Geometry check sheet. Reference: drawing and pictorial views, mm from the part's lowest x, y, z. Coordinates: 2 decimals unless noted, no trailing zeros. Order: outer loops, then holes, each group sorted by start corner. A loop starts at its lowest first (then second) coordinate and runs counter-clockwise, first axis right, second up. Notation, with made-up numbers: M 48,51.5 L 60,51.5 A8 ccw 60,55.5 Z; hole C 9.5,42.25 d7. An arc over 180 degrees is marked long. Return JSON: item names as keys, results as strings.
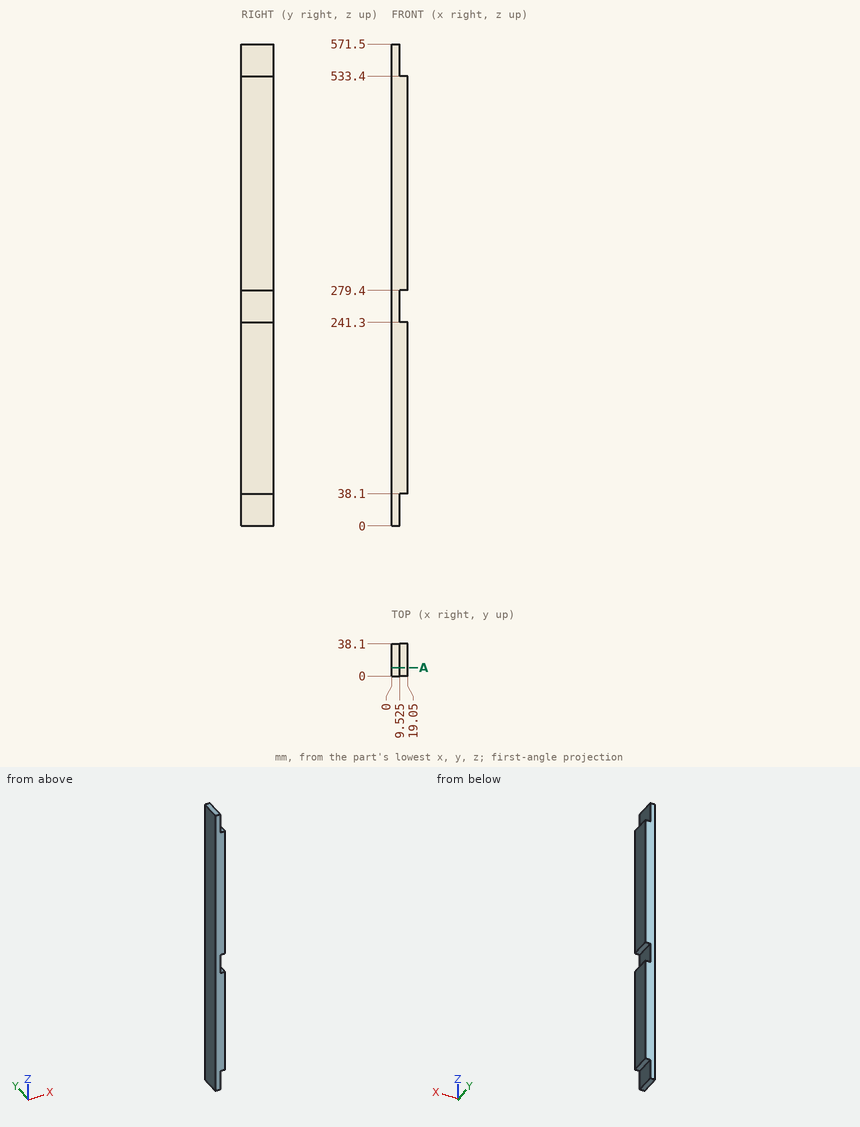
Q1. Cross-section at A-A, the plane y = 10. Record the boundary of the cut face in (x, z) (3 decimals).
Values:
{"outline": "M 0,0 L 9.525,0 L 9.525,38.1 L 19.05,38.1 L 19.05,241.3 L 9.525,241.3 L 9.525,279.4 L 19.05,279.4 L 19.05,533.4 L 9.525,533.4 L 9.525,571.5 L 0,571.5 Z"}
Q2. Go/stop test with flat-tipped pins: pin 1 (11.5 mm diameter, centred on y = 11.5, z = 556.5, fed in from +X) (3 decimals); pin 2 (3 mm diameter, centred on x = 13.5, y = 27.5, fed in from -Z); pin 3 (10.5 mm diameter, centred on x = 15, y = 24.5, fed in from +Z). Record where each tip stops, or that it passes through.
Values:
{"pin 1": "x = 9.525", "pin 2": "z = 38.1", "pin 3": "z = 533.4"}
Q3. Material ranges on line 1 along Z through (x, y) = (11, 21.5); line 2 along X through (y, z) = (16, 536.5) (3 decimals), recorded low to high.
Values:
{"line 1": "38.1 to 241.3, 279.4 to 533.4", "line 2": "0 to 9.525"}
